Part print with two shaded views. Sizes in mm from the minimum x, y, z corner. A direction names the side the tool comes from. Coordinates: 2 decimals unless noted, no trailing zeros. Loops run counter-clockwise (first coordinate to the right, second up) from the corner with the lowest first, then second, coordinate; pieces in that order, holes last.
(1) Tool access for the marked faces 4, 5, 6 and 7: list every direction of +Z, -Z, +X, -X, +Y, -Y with a clear straight run to the whole face (end or side of a thin tool).
(2) Wall check: L1, parallel to Y at x = 19.05, z = 34.25 (1 decimal); L2, parallel to Z at x = 19, y = 33.5; L3, parallel to Y at x = 22, z = 10.5 (1 decimal). Give the ranges that are in metal, low to high.
(3) Slice it at A-A (x = 19.05). Give the cut face in (y, z) (1 decimal), and give its area (3 significant figures).
(4) Two-plate mould, pull along Y, no slides. Class the marked faces 1, 2 and 3: pulls with the +Y half, pulls with the -Y half, needs draft (parallel to the pull), parting line crosses it, or undercut.
(5) Flat gauge pins, fed straight in: P1, Ø4, axis at x = 9.5, y = 26, coming from the +Z side; P2, Ø3, axis at x = 15.5, z = 23.5, coming from the -Y side (3 decimals); P3, Ø7, axis at y = 16.5, z = 7, coming from the +X side; P4, Ø8.5, axis at x = 16, y = 15, coming from the +Z side. Where does each tip first touch, or does it go through?
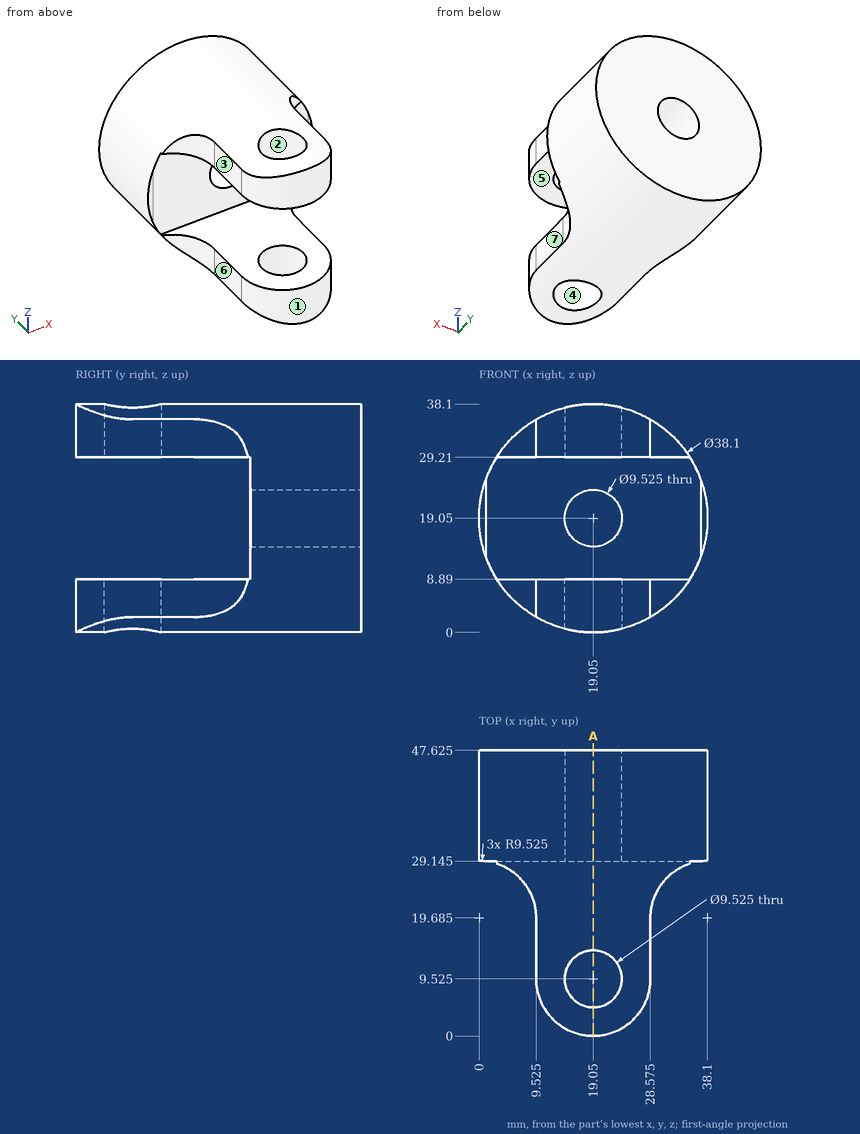
Response values:
1. face 4: +Z, -Z
1. face 5: +X, -X, -Y
1. face 6: +Z, -Z, -X, -Y
1. face 7: +Z, -Z, +X, -Y
2. L1: y = 0 to 4.8, 14.3 to 47.6
2. L2: z = 0 to 14.29, 23.81 to 38.1
2. L3: y = 29.1 to 47.6
3. outline: (0, 0) - (4.8, 0) - (4.8, 8.9) - (0, 8.9) - close; (0, 29.2) - (4.8, 29.2) - (4.8, 38.1) - (0, 38.1) - close; (14.3, 0) - (47.6, 0) - (47.6, 14.3) - (29.1, 14.3) - (29.1, 8.9) - (14.3, 8.9) - close; (14.3, 29.2) - (29.1, 29.2) - (29.1, 23.8) - (47.6, 23.8) - (47.6, 38.1) - (14.3, 38.1) - close
3. area: 877 mm2
4. face 1: pulls with the -Y half
4. face 2: undercut
4. face 3: needs draft
5. P1: stops at z = 36.54
5. P2: stops at y = 29.145
5. P3: stops at x = 28.58
5. P4: stops at z = 38.1
